The listing builds one solid part. Answer for the finished solid, in the listing's coordinates (mm). Face numbers are marked on the shaded views. A direction names the side the tool comes from. Coordinates: 2 decimals unless noted, no trailing zeros. Order: outer loops, then holes, each group sorted by start corner. A loop starts at its lowest first (then second) coordinate and runs counter-clockwise, first axis right, second up. Notation, with made-up numbers: (-24.5, 6) -> (8.5, 6) arc R25 ccw to (8.5, 22) -> close; hole circle Ø8 at (60, 6.5). An arc over 180 degrees is marked (long way). Answer in a Markdown table with one row per item. Add a question column.
```python
from build123d import *

# Parameters (mm, degrees)
SKETCH1_W           = 25.4
SKETCH1_H           = 26.924
BOSS_EXTRUDE1_DEPTH = 5.08
SKETCH2_W           = 25.4
SKETCH2_H           = 1.905
BOSS_EXTRUDE2_DEPTH = 7.62
FILLET1_R           = 7.62
SKETCH4_W           = 26.924
SKETCH4_H           = 38.735
BOSS_EXTRUDE3_DEPTH = 2.54
SKETCH6_R           = 1.27
CUT_EXTRUDE2_DEPTH  = 43.929193668
FILLET2_R           = 0.508
CUT_EXTRUDE4_DEPTH  = 49.852758377


with BuildPart() as part:
    # Sketch1 → Boss-Extrude1 (new body)
    with BuildSketch(Plane(origin=(0, 0, 0), x_dir=(1, 0, 0), z_dir=(0, 1, 0))):
        Rectangle(SKETCH1_W, SKETCH1_H)
    extrude(amount=BOSS_EXTRUDE1_DEPTH)

    # Sketch2 → Boss-Extrude2 (add)
    with BuildSketch(Plane(origin=(0, 5.08, 0), x_dir=(1, 0, 0), z_dir=(0, 1, 0))):
        with Locations((0, 12.5095)):
            Rectangle(SKETCH2_W, SKETCH2_H)
        with Locations((0, -12.5095)):
            Rectangle(SKETCH2_W, SKETCH2_H)
    extrude(amount=BOSS_EXTRUDE2_DEPTH)

    # Fillet1
    fillet1_edges = [part.edges().sort_by_distance(p)[0] for p in [
        (12.7, 12.7, -12.5095),
        (12.7, 12.7, 12.5095),
    ]]
    fillet(fillet1_edges, radius=FILLET1_R)

    # Sketch4 → Boss-Extrude3 (add)
    with BuildSketch(Plane.ZY.offset(12.7)):
        with Locations((0, 19.3675)):
            Rectangle(SKETCH4_W, SKETCH4_H)
    extrude(amount=-BOSS_EXTRUDE3_DEPTH)

    # Sketch6 → Cut-Extrude2 (cut, through all)
    with BuildSketch(Plane.XZ):
        with Locations(Location((-5.969, 0, 0), (0, 0, 270))):
            Circle(SKETCH6_R)
        with Locations(Location((0, 5.969, 0), (0, 0, 270))):
            Circle(SKETCH6_R)
        with Locations(Location((0, -5.969, 0), (0, 0, 270))):
            Circle(SKETCH6_R)
        with Locations(Location((5.969, 0, 0), (0, 0, 270))):
            Circle(SKETCH6_R)
    extrude(amount=-CUT_EXTRUDE2_DEPTH, mode=Mode.SUBTRACT)

    # Fillet2
    fillet2_edges = [part.edges().sort_by_distance(p)[0] for p in [
        (-10.16, 25.7175, -13.462),
        (-10.16, 38.735, 0),
        (-10.16, 25.7175, 13.462),
        (-12.7, 38.735, 0),
        (-12.7, 19.3675, 13.462),
        (-12.7, 19.3675, -13.462),
    ]]
    fillet(fillet2_edges, radius=FILLET2_R)

    # Sketch8 → Cut-Extrude4 (cut, through all)
    with BuildSketch(Plane(origin=(0, 0, -13.462), x_dir=(-1, 0, 0), z_dir=(0, 0, -1))):
        with BuildLine():
            ThreePointArc((-9.364, 7.08), (-7.84, 5.556), (-6.316, 7.08))
            ThreePointArc((-6.316, 7.08), (-7.84, 8.604), (-9.364, 7.08))
        make_face()
        with BuildLine():
            ThreePointArc((6.636, 7.08), (8.16, 5.556), (9.684, 7.08))
            ThreePointArc((9.684, 7.08), (8.16, 8.604), (6.636, 7.08))
        make_face()
    extrude(amount=-CUT_EXTRUDE4_DEPTH, mode=Mode.SUBTRACT)


solid = part.part
```
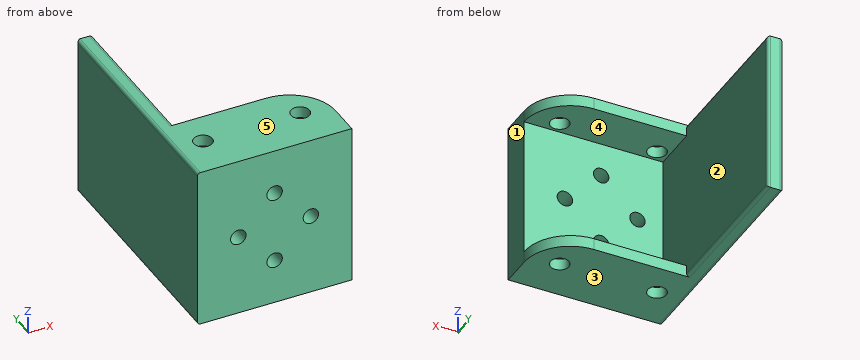
Q1. Determine the mould class of the marked faces 3, 4 and 5 for opening direction Z: +Z half, -Z half, draft (parallel to the pull), parting line (faces both ways), or undercut.
Q2. A cutting plane is placed at A-A (z = 0). Determine the outline of the cut face in (x, y) (3 decimals).
Q3. For the marked faces 1 and 2, determine the directions among +Z, -Z, +X, -X, +Y, -Y from which every point of the face is accessible in a straight line to the end or side of a thin tool.
Q4. A cutting plane is placed at C-C (y = 7.08). Determine the outline of the cut face in (x, z), then the cut area to 3 significant figures.
Q5. Given pin 1 (12 mm diameter, centred on y = 27, z = -9, fed in from +X); pin 2 (4 mm diameter, centred on x = -7, y = 19.5, fed in from -Z); pin 3 (12 mm diameter, centred on x = -0.5, z = -10, fed in from +Y), each flat-ended and moving along its own axis, determine where each tip first touches the part or whether it passes through.
Q6. A cutting plane is placed at D-D (z = 5.75). Determine the outline of the cut face in (x, y) (3 decimals), then the cut area to 3 significant figures.
Q7. Straight lines are drawn through the part: line 1 (X direction, y = 1.55, z = 0); line 2 (Z direction, x = -7.5, y = 11); line 3 (X direction, y = 18.5, z = -1.5). For each, find the intervals that lie inside material, in ascending order.
Q8. A cutting plane is placed at B-B (x = 0). Determine the outline of the cut face in (y, z).
Returned:
| question | item | result |
|---|---|---|
| 1 | face 3 | -Z half |
| 1 | face 4 | undercut |
| 1 | face 5 | +Z half |
| 2 | outline | (-12.7, 0) -> (-7.239, 0) -> (-7.239, 5.08) -> (-10.16, 5.08) -> (-10.16, 38.227) arc R0.508 ccw to (-10.668, 38.735) -> (-12.192, 38.735) arc R0.508 ccw to (-12.7, 38.227) -> close; (-4.699, 0) -> (4.699, 0) -> (4.699, 5.08) -> (-4.699, 5.08) -> close; (7.239, 0) -> (12.7, 0) -> (12.7, 5.08) -> (7.239, 5.08) -> close |
| 3 | face 1 | +Z, -Z, +X, +Y, -Y |
| 3 | face 2 | +X, +Y |
| 4 | outline | (-12.7, -12.95) arc R0.51 ccw to (-12.19, -13.46) -> (-9.68, -13.46) -> (-9.68, -11.56) -> (-10.16, -11.56) -> (-10.16, 11.56) -> (-9.68, 11.56) -> (-9.68, 13.46) -> (-12.19, 13.46) arc R0.51 ccw to (-12.7, 12.95) -> close; (-6.64, -13.46) -> (6.32, -13.46) -> (6.32, -11.56) -> (-6.64, -11.56) -> close; (-6.64, 11.56) -> (6.32, 11.56) -> (6.32, 13.46) -> (-6.64, 13.46) -> close; (9.36, -13.46) -> (12.43, -13.46) -> (12.43, -11.56) -> (9.36, -11.56) -> close; (9.36, 11.56) -> (12.43, 11.56) -> (12.43, 13.46) -> (9.36, 13.46) -> close |
| 4 | area | 131 mm² |
| 5 | pin 1 | stops at x = -10.16 |
| 5 | pin 2 | passes through |
| 5 | pin 3 | stops at y = 12.7 |
| 6 | outline | (-12.7, 0) -> (-1.251, 0) -> (-1.251, 5.08) -> (-10.16, 5.08) -> (-10.16, 38.227) arc R0.508 ccw to (-10.668, 38.735) -> (-12.192, 38.735) arc R0.508 ccw to (-12.7, 38.227) -> close; (1.251, 0) -> (12.7, 0) -> (12.7, 5.08) -> (1.251, 5.08) -> close |
| 6 | area | 202 mm² |
| 7 | line 1 | x = -12.7 to -7.24, -4.7 to 4.7, 7.24 to 12.7 |
| 7 | line 2 | z = -13.46 to -11.56, 11.56 to 13.46 |
| 7 | line 3 | x = -12.7 to -10.16 |
| 8 | outline | (0, -13.46) -> (12.7, -13.46) -> (12.7, -11.56) -> (5.08, -11.56) -> (5.08, -7.24) -> (0, -7.24) -> close; (0, -4.7) -> (5.08, -4.7) -> (5.08, 4.7) -> (0, 4.7) -> close; (0, 7.24) -> (5.08, 7.24) -> (5.08, 11.56) -> (12.7, 11.56) -> (12.7, 13.46) -> (0, 13.46) -> close |
